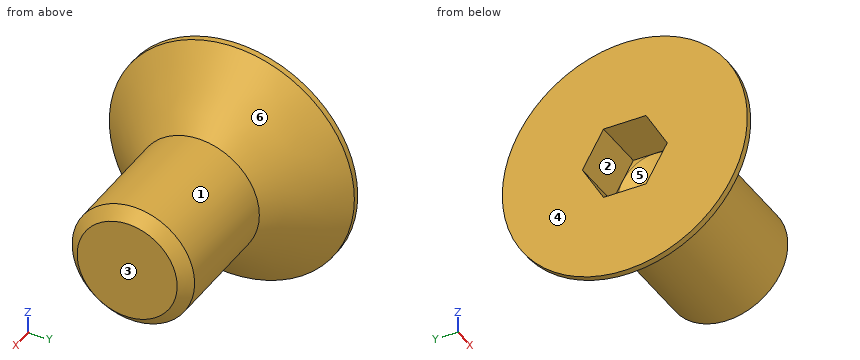
Autodesk Inventor part; units mm, degrees
ref_plane "screw_to_nut_XY" through (0, 0, 0) normal (1, 0, 0) x (0, 0, -1)
ref_plane "screw_to_nut_YZ" through (0, 0, 0) normal (0, 0, -1) x (0, 1, 0)
ref_plane "screw_to_nut_ZX" through (0, 0, 0) normal (0, 1, 0) x (1, 0, 0)
sketch "Sketch_1" plane through (0, 0, 0) normal (0, 0, 1) x (1, 0, 0)
  line L0 (16, 0) -> (0, 0)
  line L1 (0, 0) -> (0, 10)
  line L2 (0, 10) -> (0.5, 10)
  line L3 (0.5, 10) -> (5.5, 5)
  line L4 (5.5, 5) -> (15.08, 5)
  line L5 (15.08, 5) -> (16, 4.08)
  line L6 (16, 4.08) -> (16, 0)
  line L7 (16, 0) -> (0, 0)
revolve "Revolution1" add sketch "Sketch_1" angle 360 about axis through (16, 0, 0) along (1, 0, 0)
thread "Thread1"
sketch "Sketch2" plane through (0, 0, 0) normal (-1, 0, 0) x (0, 0, 1)
  point P0 (0, 0)
hole "Hole1" at (0, 0, 0) direction (1, 0, 0) diameter 6 depth 4.4 tip angle 150
sketch "Sketch_3" plane through (0, 0, 0) normal (1, 0, 0) x (0, 1, 0)
  line L0 (-1.7321, 3) -> (-3.4641, 0)
  line L1 (-3.4641, 0) -> (-1.7321, -3)
  line L2 (-1.7321, -3) -> (1.7321, -3)
  line L3 (1.7321, -3) -> (3.4641, 0)
  line L4 (3.4641, 0) -> (1.7321, 3)
  line L5 (1.7321, 3) -> (-1.7321, 3)
extrude "Extrusion1" cut sketch "Sketch_3" along normal blind 4.4
ref_plane "screw_to_nut_XY" through (0, 0, 0) normal (1, 0, 0) x (0, 0, -1)
ref_plane "screw_to_nut_YZ" through (0, 0, 0) normal (0, 0, -1) x (0, 1, 0)
ref_plane "screw_to_nut_ZX" through (0, 0, 0) normal (0, 1, 0) x (1, 0, 0)
properties part number "FB10-16_"
Design review of the part built by this model. Coordinates are the model's own, in mm. Face numbers are marked on the shaded views. A direction names the side the tool comes from. Give positions to 0.01 mm unless a question says otherwise; leave off trailing zeros. Order: outer loops, then holes, each group sorted by start corner. A loop starts at its lowest first (then second) coordinate and runs counter-clockwise, first axis right, second up.
1. To check wall thickness, follow L1, parallel to X at y = 6, z = 4.5; L2, parallel to Y at x = 14, z = -0.25; L3, parallel to Z at x = 10, y = -1.25. State the ranges of each line that lie inside material, in increasing order.
Solution:
L1: x = 0 to 3
L2: y = -4.99 to 4.99
L3: z = -4.84 to 4.84
2. Tool access review of the marked faces 1, 2 and 3: name each direction out of +Z, -Z, +X, -X, +Y, -Y from which nothing blocks a thin tool from reaching the whole face with its end or side.
Solution:
face 1: +X
face 2: -X
face 3: +Z, -Z, +X, +Y, -Y
3. Mouldability with a two-part tool opening along Y and no side actions: class the marked faces 4, 5 and 6 as +Y half, -Y half, draft (parallel to the pull), parting line (faces both ways), or undercut.
Solution:
face 4: draft
face 5: undercut
face 6: parting line
4. Add section A-A, the plane x = 3. State the section outline as (y, z) points, then the cut area to 3 significant figures.
Solution:
outline: circle Ø15 at (0, 0); hole (-3.46, 0) - (-1.73, -3) - (1.73, -3) - (3.46, 0) - (1.73, 3) - (-1.73, 3) - close
area: 146 mm2
5. Add section B-B, the plane x = 14.25. State the section outline as (y, z) points.
Solution:
outline: circle Ø10 at (0, 0)
6. For pin 1 Ø1 at (y, z) = (6.5, 4) entering from +X; pin 2 Ø5 at (x, z) = (7, -0.5) entering from +Y; pin 3 Ø1.7 at (x, y) = (2, -0.5) entering from +Z, all flat-tipped, find the tip position at first contact; note any pin that passes through.
Solution:
pin 1: stops at x = 3.37
pin 2: stops at y = 5.99
pin 3: stops at z = 9.34
